```python
from build123d import *

# Parameters (mm, degrees)
BOSS_EXTRUDE1_DEPTH = 3
CUT_EXTRUDE1_DEPTH  = 6
SKETCH4_W           = 12
SKETCH4_H           = 6
SKETCH4_W_2         = 55
SKETCH4_W_3         = 5
SKETCH4_W_4         = 6
SKETCH4_H_2         = 4
CUT_EXTRUDE2_DEPTH  = 6
CUT_EXTRUDE3_REACH  = 8
SKETCH5_W           = 20
SKETCH5_H           = 6


with BuildPart() as part:
    # Sketch1 → Boss-Extrude1 (new body, symmetric)
    with BuildSketch(Plane(origin=(0, 0, 0), x_dir=(0, 0, -1), z_dir=(1, 0, 0))):
        Polygon((0, 0), (250, 0), (250, 65), (60, 65), (0, 65), align=None)
    extrude(amount=BOSS_EXTRUDE1_DEPTH, both=True)

    # Sketch3 → Cut-Extrude1 (cut)
    with BuildSketch(Plane(origin=(3, 0, 0), x_dir=(0, 0, -1), z_dir=(1, 0, 0))):
        with BuildLine():
            Line((0, 0), (88, 0))
            Line((88, 0), (88, 45))
            ThreePointArc((88, 45), (85.071067812, 52.071067812), (78, 55))
            Line((78, 55), (0, 55))
            Line((0, 55), (0, 0))
        make_face()
    extrude(amount=-CUT_EXTRUDE1_DEPTH, mode=Mode.SUBTRACT)

    # Sketch4 → Cut-Extrude2 (cut)
    with BuildSketch(Plane(origin=(3, 0, 0), x_dir=(0, 0, -1), z_dir=(1, 0, 0))):
        with Locations((94, 3)):
            Rectangle(SKETCH4_W, SKETCH4_H)
        with Locations((167.5, 3)):
            Rectangle(SKETCH4_W_2, SKETCH4_H)
        with Locations((247.5, 3)):
            Rectangle(SKETCH4_W_3, SKETCH4_H)
        Polygon((245, 16), (250, 16), (250, 65), (239, 65), (239, 16), align=None)
        with Locations((8, 57)):
            Rectangle(SKETCH4_W_4, SKETCH4_H_2)
    extrude(amount=-CUT_EXTRUDE2_DEPTH, mode=Mode.SUBTRACT)

    # Sketch5 → Cut-Extrude3 (cut, up to next)
    with BuildSketch(Plane(origin=(3, 0, 0), x_dir=(0, 0, -1), z_dir=(1, 0, 0)), mode=Mode.PRIVATE) as cut_extrude3_sk1:
        with Locations((169, 62)):
            Rectangle(SKETCH5_W, SKETCH5_H)
    cut_extrude3_tool1 = extrude(cut_extrude3_sk1.sketch, amount=-CUT_EXTRUDE3_REACH, mode=Mode.PRIVATE) & part.part
    add(cut_extrude3_tool1.solids().sort_by_distance((3, 62, -169))[0], mode=Mode.SUBTRACT)
    # Sketch5 → Cut-Extrude3 (cut, up to next)
    with BuildSketch(Plane(origin=(3, 0, 0), x_dir=(0, 0, -1), z_dir=(1, 0, 0)), mode=Mode.PRIVATE) as cut_extrude3_sk2:
        with Locations((209, 62)):
            Rectangle(SKETCH5_W, SKETCH5_H)
    cut_extrude3_tool2 = extrude(cut_extrude3_sk2.sketch, amount=-CUT_EXTRUDE3_REACH, mode=Mode.PRIVATE) & part.part
    add(cut_extrude3_tool2.solids().sort_by_distance((3, 62, -209))[0], mode=Mode.SUBTRACT)
    # Sketch5 → Cut-Extrude3 (cut, up to next)
    with BuildSketch(Plane(origin=(3, 0, 0), x_dir=(0, 0, -1), z_dir=(1, 0, 0)), mode=Mode.PRIVATE) as cut_extrude3_sk3:
        with Locations((129, 62)):
            Rectangle(SKETCH5_W, SKETCH5_H)
    cut_extrude3_tool3 = extrude(cut_extrude3_sk3.sketch, amount=-CUT_EXTRUDE3_REACH, mode=Mode.PRIVATE) & part.part
    add(cut_extrude3_tool3.solids().sort_by_distance((3, 62, -129))[0], mode=Mode.SUBTRACT)
    # Sketch5 → Cut-Extrude3 (cut, up to next)
    with BuildSketch(Plane(origin=(3, 0, 0), x_dir=(0, 0, -1), z_dir=(1, 0, 0)), mode=Mode.PRIVATE) as cut_extrude3_sk4:
        with Locations((89, 62)):
            Rectangle(SKETCH5_W, SKETCH5_H)
    cut_extrude3_tool4 = extrude(cut_extrude3_sk4.sketch, amount=-CUT_EXTRUDE3_REACH, mode=Mode.PRIVATE) & part.part
    add(cut_extrude3_tool4.solids().sort_by_distance((3, 62, -89))[0], mode=Mode.SUBTRACT)
    # Sketch5 → Cut-Extrude3 (cut, up to next)
    with BuildSketch(Plane(origin=(3, 0, 0), x_dir=(0, 0, -1), z_dir=(1, 0, 0)), mode=Mode.PRIVATE) as cut_extrude3_sk5:
        with Locations((49, 62)):
            Rectangle(SKETCH5_W, SKETCH5_H)
    cut_extrude3_tool5 = extrude(cut_extrude3_sk5.sketch, amount=-CUT_EXTRUDE3_REACH, mode=Mode.PRIVATE) & part.part
    add(cut_extrude3_tool5.solids().sort_by_distance((3, 62, -49))[0], mode=Mode.SUBTRACT)


solid = part.part
```
Input: part model. Units: mm. Frame: model coordinates. A direction names the side the tool comes from. Give positions to 0.01 mm unless a question says otherwise; leave off trailing zeros. Loops run counter-clockwise (first coordinate to the right, second up) from the corner with the lowest first, then second, coordinate; pieces in that order, holes last.
1) Section query A-A on y = 40. Return the cut outline in (x, z).
A:
outline: (-3, -239) - (3, -239) - (3, -88) - (-3, -88) - close
2) Reachability of faces 1 (the flat face through (0, 62, -159)), 2 (the flat face through (0, 11, -250)), 3 (the flat face through (0, 3, -100)), 4 (the flat face through (0, 0, -120)), 5 (the flat face through (0, 59, -8)) from +Z, -Z, +X, -X, +Y, -Y: full face, straight path, thin tool, end or side. Return the list, or none.
A:
face 1: +X, -X, +Y
face 2: -Z, +X, -X, +Y, -Y
face 3: +Z, +X, -X, -Y
face 4: +Z, -Z, +X, -X, -Y
face 5: +X, -X, -Y
3) Mould query, pull axis Z, two halves, no side actions, for faces 6 (the flat face through (0, 60, 0)), 7 (the flat face through (0, 59, -49)), 8 (the flat face through (0, 6, -247)), 9 (the flat face through (0, 57, -5)). Classes: released by +Z, released by -Z, zero draft, split by the parting line, or undercut.
A:
face 6: released by +Z
face 7: undercut
face 8: zero draft
face 9: undercut
4) Contact query for flat-ended pins moving along their axis: pin 1 (3 mm diameter, centred on x = 1, y = 61.5, fed in from +Z); pin 2 (3 mm diameter, centred on x = 0, y = 2.5, fed in from -Z); pin 3 (1.5 mm diameter, centred on x = 2, y = 42, fed in from +Z); pin 4 (1.8 mm diameter, centred on x = 0.5, z = -244.5, fed in from +Y). Output: stop coordinate, or through.
A:
pin 1: stops at z = 0
pin 2: stops at z = -245
pin 3: stops at z = -88
pin 4: stops at y = 16
5) Section query B-B on z = -62. Return the cut outline in (x, y).
A:
outline: (-3, 55) - (3, 55) - (3, 65) - (-3, 65) - close
6) Line query: L1, parallel to Z at x = -1.45, y = 61; L2, parallel to Z at x = 1.95, y = 4; L3, parallel to Y at x = -0.15, z = -66. Output: solid intervals per line, ascending.
A:
L1: z = -239 to -219, -199 to -179, -159 to -139, -119 to -99, -79 to -59, -39 to 0
L2: z = -245 to -195, -140 to -100
L3: y = 55 to 65
